Check sheet for the modelled part. Datum: model origin and axes. Units: mm. Face numbers are marked on the shaded views. Round coordinates to 2 decimals unless told otherwise and drop trailing zeros. Order: outer loops, then holes, each group sorted by start corner. A loop starts at its lowest first (then second) coordinate and runs counter-clockwise, first axis right, second up.
```python
from build123d import *

# Parameters (mm, degrees)
F0_R     = 25.4
F1_DEPTH = 76.2
F2_R     = 22.225
F3_DEPTH = 69.85
F4_R     = 5.08
F5_R     = 2.54
F6_R     = 1.27


with BuildPart() as f1:
    # F0 (on Top) → F1 (new body)
    with BuildSketch(Plane.XY):
        Circle(F0_R)
    extrude(amount=F1_DEPTH)

    # F2 (on face) → F3 (cut)
    with BuildSketch(Plane.XY.offset(76.2)):
        Circle(F2_R)
    extrude(amount=-F3_DEPTH, mode=Mode.SUBTRACT)

    # F4
    f4_edges = [f1.edges().sort_by_distance(p)[0] for p in [
        (-22.225, 0, 6.35),
    ]]
    fillet(f4_edges, radius=F4_R)

    # F5
    f5_edges = [f1.edges().sort_by_distance(p)[0] for p in [
        (-25.4, 0, 76.2),
    ]]
    fillet(f5_edges, radius=F5_R)

    # F6
    f6_edges = [f1.edges().sort_by_distance(p)[0] for p in [
        (-25.4, 0, 0),
    ]]
    fillet(f6_edges, radius=F6_R)


solid = f1.part
```
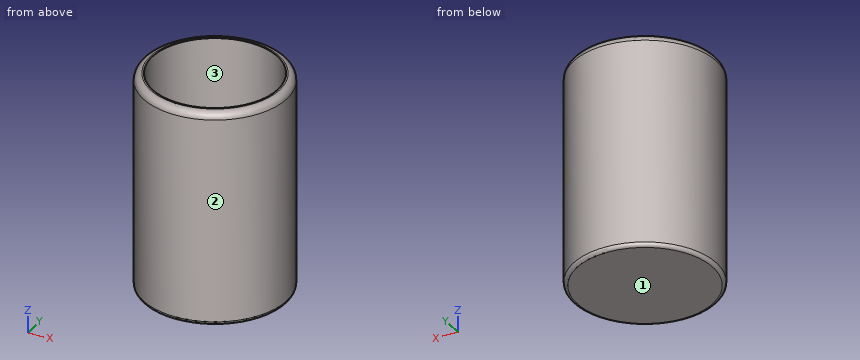
Item 1: Sectioned sample at A-A (z = 41.5). Record the cut outline in (x, y) (3 decimals).
Answer:
outline: circle Ø50.8 at (0, 0); hole circle Ø44.45 at (0, 0)
Item 2: Sectioned sample at B-B (y = 0). Record the cut outline in (x, z) (3 decimals), and give its area (3 significant figures).
Answer:
outline: (-25.4, 1.27) arc R1.27 ccw to (-24.13, 0) - (24.13, 0) arc R1.27 ccw to (25.4, 1.27) - (25.4, 73.66) arc R2.54 ccw to (22.86, 76.2) - (22.225, 76.2) - (22.225, 11.43) arc R5.08 cw to (17.145, 6.35) - (-17.145, 6.35) arc R5.08 cw to (-22.225, 11.43) - (-22.225, 76.2) - (-22.86, 76.2) arc R2.54 ccw to (-25.4, 73.66) - close
area: 774 mm2
Item 3: Release check for a two-part mould opening along Y. For the marked faces 1, 2 and 3 record: released by +Y, released by -Y, zero draft, split by the parting line, or undercut.
Answer:
face 1: zero draft
face 2: split by the parting line
face 3: undercut
Item 4: Go/stop test with flat-tipped pins: P1, Ø10, axis at x = 13, y = -6.5, coming from the +Z side; P2, Ø4, axis at y = -8.5, z = 27, coming from the +X side; P3, Ø1, axis at x = 19.5, y = 13.5, coming from the +Z side. Record where each tip stops, or that it passes through.
Answer:
P1: stops at z = 6.95
P2: stops at x = 24.55
P3: stops at z = 76.17
Item 5: Sectioned sample at D-D (z = 5.5). Record the cut outline in (x, y).
Answer:
outline: circle Ø50.8 at (0, 0)
Item 6: Scan lines: line 1 along Y through (x, z) = (0, 48) (3 decimals); line 2 along Z through (x, y) = (8.5, -14); line 3 along Z through (x, y) = (-0.5, -23). Record each from-to range of solid material in increasing order.
Answer:
line 1: y = -25.4 to -22.225, 22.225 to 25.4
line 2: z = 0 to 6.35
line 3: z = 0 to 76.2
